Source: CAD feature listing. Evaluate the final solid. Frame: model axes, mm. Face numbers are marked on the shaded views. A direction names the side the tool comes from. Give positions to 0.01 mm unless a question says otherwise; leave off trailing zeros. Order: outer loops, then holes, each group sorted by start corner. A loop starts at its lowest first (then second) coordinate and runs counter-clockwise, first axis right, second up.
1) Section C-C, the plane z = 10.25. Return loops of the section in (x, y).
2) Draft query along Z for the marked faces 1, 2, 3 and 4. Return one class per face: released by +Z, released by -Z, zero draft, split by the parting line, or undercut.
3) First-contact query: P1, Ø4, axis at x = 3.5, z = 1, coming from the -Y side; P2, Ø1.5, axis at y = -2, z = 6.5, coming from the -X side; P3, Ø5, axis at x = 2, z = 9, coming from the -Y side; P4, Ø1, axis at x = 13, z = 7.5, coming from the +Y side. Flat tips, straight axial feed; report the tip coordinate or a pass-through.
4) Section B-B, the plane y = -1. Return loops of the section in (x, z), plus the area to 3 significant figures.
5) Section D-D, the plane y = 5. Return loops of the section in (x, z), plus the area to 3 significant figures.
6) Section A-A, the plane x = 12.7. Return loops of the section in (y, z).
7) Material intervals for line 1 (Z direction, x = 10.5, y = -4.25); line 2 (Y direction, x = 12.7, z = 8.5); line 3 (X direction, y = -1.75, z = 5.5), sorted ascending.
8) Access query for the marked faces 5 and 6. Directions: +Z, -Z, +X, -X, +Y, -Y. A direction counts if a zero-diameter tool reaches every point of the face in a straight line with its end or side. Return the directions, or none.
```python
from build123d import *

# Parameters (mm, degrees)
BOSS_EXTRUDE1_DEPTH = 1.5
SKETCH2_R           = 3.96
BOSS_EXTRUDE2_DEPTH = 7.95
SKETCH3_R           = 2
CUT_EXTRUDE1_DEPTH  = 23.321010282


with BuildPart() as part:
    # Sketch1 → Boss-Extrude1 (new body)
    with BuildSketch(Plane.XY):
        with BuildLine():
            ThreePointArc((2.081092437, 5.467316917), (-5.85, 0), (2.081092437, -5.467316917))
            ThreePointArc((2.081092437, -5.467316917), (6.35, -4.682325977), (10.618907563, -5.467316917))
            ThreePointArc((10.618907563, -5.467316917), (18.55, 0), (10.618907563, 5.467316917))
            ThreePointArc((10.618907563, 5.467316917), (6.35, 4.682325977), (2.081092437, 5.467316917))
        make_face()
    extrude(amount=BOSS_EXTRUDE1_DEPTH)


with BuildPart() as body_2:
    # Mirror2: mirrored copy
    add(part.part.mirror(Plane.XY.offset(5.475)))


with BuildPart() as part_1:
    add(part.part)

    add(body_2.part)  # Boss-Extrude2 merges body 2
    # Sketch2 → Boss-Extrude2 (add)
    with BuildSketch(Plane.XY.offset(1.5)):
        with Locations(Location((0, 0, 0), (0, 0, 180))):
            Circle(SKETCH2_R)
        with Locations(Location((12.7, 0, 0), (0, 0, 180))):
            Circle(SKETCH2_R)
    extrude(amount=BOSS_EXTRUDE2_DEPTH)

    # Sketch3 → Cut-Extrude1 (cut, through all)
    with BuildSketch(Plane(origin=(0, 0, 0), x_dir=(-1, 0, 0), z_dir=(0, 0, -1))):
        Circle(SKETCH3_R)
        with Locations((-12.7, 0)):
            Circle(SKETCH3_R)
    extrude(amount=-CUT_EXTRUDE1_DEPTH, mode=Mode.SUBTRACT)


solid = part_1.part
```
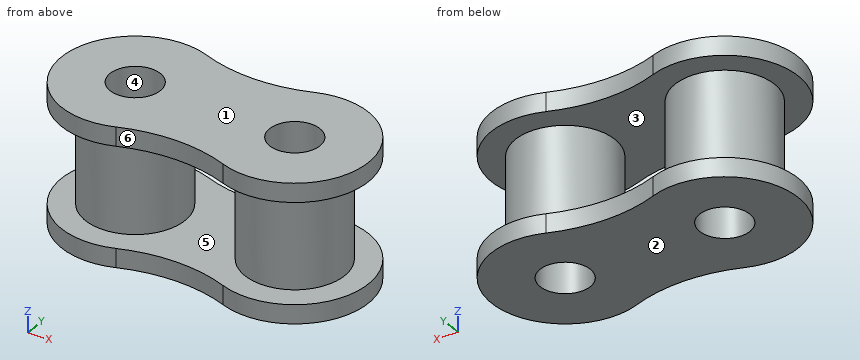
From the geometry:
1. outline: (2.08, -5.47) arc R12 cw to (10.62, -5.47) arc R5.85 ccw (long way) to (10.62, 5.47) arc R12 cw to (2.08, 5.47) arc R5.85 ccw (long way) to start; hole circle Ø4 at (0, 0); hole circle Ø4 at (12.7, 0)
2. face 1: released by +Z
2. face 2: released by -Z
2. face 3: undercut
2. face 4: zero draft
3. P1: stops at y = -5.65
3. P2: stops at x = -3.76
3. P3: stops at y = -5.85
3. P4: stops at y = 3.96
4. outline: (-5.76, 0) - (-1.73, 0) - (-1.73, 10.95) - (-5.76, 10.95) - (-5.76, 9.45) - (-3.83, 9.45) - (-3.83, 1.5) - (-5.76, 1.5) - close; (1.73, 0) - (10.97, 0) - (10.97, 10.95) - (1.73, 10.95) - close; (14.43, 0) - (18.46, 0) - (18.46, 1.5) - (16.53, 1.5) - (16.53, 9.45) - (18.46, 9.45) - (18.46, 10.95) - (14.43, 10.95) - close; hole (3.83, 1.5) - (8.87, 1.5) - (8.87, 9.45) - (3.83, 9.45) - close
4. area: 119 mm2
5. outline: (-3.04, 0) - (3.61, 0) - (3.61, 1.5) - (-3.04, 1.5) - close; (-3.04, 9.45) - (3.61, 9.45) - (3.61, 10.95) - (-3.04, 10.95) - close; (9.09, 0) - (15.74, 0) - (15.74, 1.5) - (9.09, 1.5) - close; (9.09, 9.45) - (15.74, 9.45) - (15.74, 10.95) - (9.09, 10.95) - close
5. area: 39.9 mm2
6. outline: (-5.85, 0) - (-2, 0) - (-2, 10.95) - (-5.85, 10.95) - (-5.85, 9.45) - (-3.96, 9.45) - (-3.96, 1.5) - (-5.85, 1.5) - close; (2, 0) - (5.85, 0) - (5.85, 1.5) - (3.96, 1.5) - (3.96, 9.45) - (5.85, 9.45) - (5.85, 10.95) - (2, 10.95) - close
7. line 1: z = 0 to 1.5, 9.45 to 10.95
7. line 2: y = -3.96 to -2, 2 to 3.96
7. line 3: x = -3.55 to -0.97, 0.97 to 3.55, 9.15 to 11.73, 13.67 to 16.25
8. face 5: none
8. face 6: +Z, -Z, -Y
